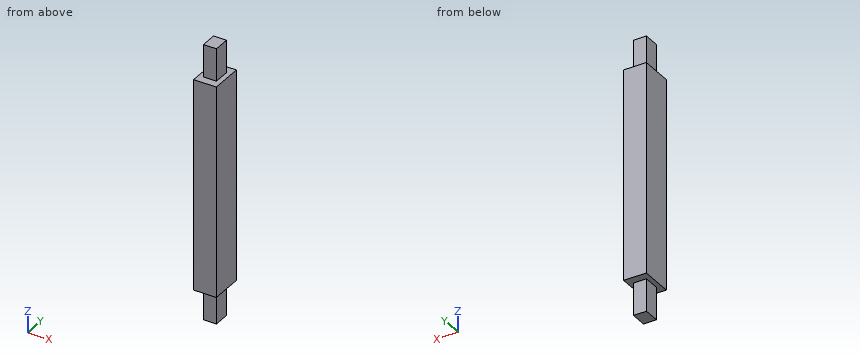
```python
from build123d import *

# Parameters (mm, degrees)
SKETCH1_W           = 7
SKETCH1_H           = 10
BOSS_EXTRUDE1_DEPTH = 32.5
SKETCH2_W           = 4
SKETCH2_H           = 5
BOSS_EXTRUDE2_DEPTH = 10
SKETCH3_W           = 4
SKETCH3_H           = 5
BOSS_EXTRUDE3_DEPTH = 10


with BuildPart() as part:
    # Sketch1 → Boss-Extrude1 (new body, symmetric)
    with BuildSketch(Plane.XY):
        Rectangle(SKETCH1_W, SKETCH1_H)
    extrude(amount=BOSS_EXTRUDE1_DEPTH, both=True)

    # Sketch2 → Boss-Extrude2 (add)
    with BuildSketch(Plane.XY.offset(32.5)):
        Rectangle(SKETCH2_W, SKETCH2_H)
    extrude(amount=BOSS_EXTRUDE2_DEPTH)

    # Sketch3 → Boss-Extrude3 (add)
    with BuildSketch(Plane(origin=(0, 0, -32.5), x_dir=(-1, 0, 0), z_dir=(0, 0, -1))):
        Rectangle(SKETCH3_W, SKETCH3_H)
    extrude(amount=BOSS_EXTRUDE3_DEPTH)


solid = part.part
```
Geometry: final body of the model. Coordinates: model frame, mm. Coordinates: 2 decimals unless noted, no trailing zeros. Loops run counter-clockwise (first coordinate to the right, second up) from the corner with the lowest first, then second, coordinate; pieces in that order, holes last. Notation, with made-up numbers: (-4, 19) -> (40, 19) arc R10 ccw to (40, 25) -> close; hole circle Ø7 at (1.5, 10). An arc over 180 degrees is marked (long way). Use a Markdown table: item, result. Add a question column.
(1) Section query C-C, the plane z = 35. Return loops of the section in (x, y), plus the area to 3 significant figures.
(2) Section query A-A, the plane x = -0.5. Return loops of the section in (y, z).
(3) Pin query (flat end, axial travel): pin 1 Ø2 at (x, z) = (0, -35.5) entering from -Y; pin 2 Ø2 at (x, z) = (0.5, -36.5) entering from +Y; pin 3 Ø4 at (y, z) = (-0.5, -35.5) entering from +X. Return the tip coordinate at first contact, or that it passes through.
(4) Section query B-B, the plane y = 1.25. Return loops of the section in (x, z), plus the area to 3 significant figures.
(5) Line query: line 1 along Z through (x, y) = (0.5, -4); line 2 along Y through (x, z) = (-1, 38). Output: solid intervals per line, ascending.
Answer:
| question | item | result |
|---|---|---|
| 1 | outline | (-2, -2.5) -> (2, -2.5) -> (2, 2.5) -> (-2, 2.5) -> close |
| 1 | area | 20.0 mm^2 |
| 2 | outline | (-5, -32.5) -> (-2.5, -32.5) -> (-2.5, -42.5) -> (2.5, -42.5) -> (2.5, -32.5) -> (5, -32.5) -> (5, 32.5) -> (2.5, 32.5) -> (2.5, 42.5) -> (-2.5, 42.5) -> (-2.5, 32.5) -> (-5, 32.5) -> close |
| 3 | pin 1 | stops at y = -2.5 |
| 3 | pin 2 | stops at y = 2.5 |
| 3 | pin 3 | stops at x = 2 |
| 4 | outline | (-3.5, -32.5) -> (-2, -32.5) -> (-2, -42.5) -> (2, -42.5) -> (2, -32.5) -> (3.5, -32.5) -> (3.5, 32.5) -> (2, 32.5) -> (2, 42.5) -> (-2, 42.5) -> (-2, 32.5) -> (-3.5, 32.5) -> close |
| 4 | area | 535 mm^2 |
| 5 | line 1 | z = -32.5 to 32.5 |
| 5 | line 2 | y = -2.5 to 2.5 |
